Autodesk Inventor part; units mm, degrees
ref_plane "YZ Plane" through (0, 0, 0) normal (1, 0, 0) x (0, 1, 0)
ref_plane "XZ Plane" through (0, 0, 0) normal (0, 1, 0) x (-1, 0, 0)
ref_plane "XY Plane" through (0, 0, 0) normal (0, 0, 1) x (1, 0, 0)
sketch "スケッチ1" plane through (0, 0, 0) normal (0, 0, 1) x (1, 0, 0)
  line L0 (-20.6499, 10.2438) -> (19.8501, 10.2438)
  line L1 (19.8501, 10.2438) -> (19.8501, -10.7562)
  line L2 (19.8501, -10.7562) -> (-20.6499, -10.7562)
  line L3 (-20.6499, -10.7562) -> (-20.6499, 10.2438)
  dimension "d0" = 21
  dimension "d1" = 40.5
extrude "押し出し1" add sketch "スケッチ1" along normal blind 41.8
sketch "スケッチ2" plane through (0, 0, 41.8) normal (0, 0, 1) x (1, 0, 0)
  line L0 (-20.6499, 10.2438) -> (19.8501, 10.2438)
  line L1 (-20.6499, -10.7562) -> (-20.6499, 10.2438)
  line L2 (-13.3999, 16.2438) -> (12.6001, 16.2438)
  line L3 (12.6001, 16.2438) -> (12.6001, -16.7562)
  line L4 (12.6001, -16.7562) -> (-13.3999, -16.7562)
  line L5 (-13.3999, -16.7562) -> (-13.3999, 16.2438)
  line L6 (-13.3999, 12.7438) -> (12.6001, 12.7438)
  line L7 (12.6001, 12.7438) -> (12.6001, -13.2562)
  line L8 (12.6001, -13.2562) -> (-13.3999, -13.2562)
  line L9 (-13.3999, -13.2562) -> (-13.3999, 12.7438)
  circle A0 centre (-13.3999, 12.7438) radius 3.5
  circle A1 centre (-13.3999, -13.2562) radius 3.5
  circle A2 centre (12.6001, -13.2562) radius 3.5
  circle A3 centre (12.6001, 12.7438) radius 3.5
  line L10 (-16.8999, 12.7438) -> (-9.8999, 12.7438)
  line L11 (-9.8999, 12.7438) -> (-9.8999, -13.2562)
  line L12 (-9.8999, -13.2562) -> (-16.8999, -13.2562)
  line L13 (-16.8999, -13.2562) -> (-16.8999, 12.7438)
  line L14 (9.1001, 12.7438) -> (16.1001, 12.7438)
  line L15 (16.1001, 12.7438) -> (16.1001, -13.2562)
  line L16 (16.1001, -13.2562) -> (9.1001, -13.2562)
  line L17 (9.1001, -13.2562) -> (9.1001, 12.7438)
  dimension "d4" = 6
  dimension "d5" = 33
  dimension "d6" = 26
  dimension "d7" = 7.25
  dimension "d8" = 26
  dimension "d9" = 2.5
  dimension "d10" = 26
  dimension "d11" = 7
  dimension "d12" = 7
  dimension "d13" = 7
  dimension "d14" = 7
extrude "押し出し2" add sketch "スケッチ2" against normal blind 3.7 contours L13 A0 L0 | L0 A0 L5 A1 L13 | A0 L10 L5 L0 | L0 L5 A0 | L12 L5 A1 | A1 L5 L12 | A0 L5 L10 | L5 L6 A0 L0 | L0 A0 L5 | A0 L0 L11 A1 L5 | L5 L8 A1 | A1 L8 L5 | A0 L6 L5 | A0 L11 L0 | A2 L8 L3 | L3 L16 A2 | A3 L14 L3 | L3 L6 A3 | L8 A2 L3 | L3 A2 L16 | L17 L0 A3 L3 A2 | A2 L3 A3 L0 L15 | L14 A3 L0 L3 | L3 L0 A3 L6 | L15 L0 A3 | A3 L0 L17 | L3 A3 L0 | L0 A3 L3
sketch "スケッチ3" plane through (0, 0, 41.8) normal (0, 0, 1) x (1, 0, 0)
  line L0 (-20.6499, -10.7562) -> (-20.6499, 10.2438)
  line L1 (-9.8999, 10.2438) -> (9.1001, 10.2438)
  circle A0 centre (9.5501, -0.2562) radius 4
  dimension "d17" = 10.5
  dimension "d18" = 30.2
  dimension "d19" = 8
extrude "押し出し3" add sketch "スケッチ3" along normal blind 1.9
sketch "スケッチ4" plane through (9.5501, -0.2562, 43.7) normal (0, 0, 1) x (1, 0, 0)
  circle A0 centre (0, 0) radius 4
  circle A1 centre (0, 0) radius 10.5
  dimension "d22" = 21
extrude "押し出し4" add sketch "スケッチ4" along normal blind 1.9 contours A0 | A1
sketch "スケッチ5" plane through (9.5501, -0.2562, 45.6) normal (0, 0, 1) x (1, 0, 0)
  circle A0 centre (0, 0) radius 10.5
  circle A1 centre (0, 0) radius 4
  dimension "d25" = 8
extrude "押し出し5" add sketch "スケッチ5" along normal blind 1.2 contours A1
sketch "スケッチ6" plane through (9.5501, -0.2562, 46.8) normal (0, 0, 1) x (1, 0, 0)
  circle A0 centre (0, 0) radius 4
  circle A1 centre (0, 0) radius 2.75
  dimension "d28" = 5.5
extrude "押し出し6" add sketch "スケッチ6" along normal blind 3 contours A1
sketch "スケッチ7" plane through (0, 0, 0) normal (0, 0, -1) x (-1, 0, 0)
  line L0 (9.8999, -10.7562) -> (16.8999, -10.7562)
  line L1 (9.8999, -13.2562) -> (9.8999, -10.7562)
  arc A0 (9.8999, -13.2562) -> (16.8999, -13.2562) centre (13.3999, -13.2562) ccw
  line L2 (16.8999, -10.7562) -> (16.8999, -13.2562)
  line L3 (16.8999, 10.2438) -> (9.8999, 10.2438)
  line L4 (16.8999, 12.7438) -> (16.8999, 10.2438)
  arc A1 (16.8999, 12.7438) -> (9.8999, 12.7438) centre (13.3999, 12.7438) ccw
  line L5 (9.8999, 10.2438) -> (9.8999, 12.7438)
  line L6 (-9.1001, 10.2438) -> (-16.1001, 10.2438)
  line L7 (-9.1001, 12.7438) -> (-9.1001, 10.2438)
  arc A2 (-9.1001, 12.7438) -> (-16.1001, 12.7438) centre (-12.6001, 12.7438) ccw
  line L8 (-16.1001, 10.2438) -> (-16.1001, 12.7438)
  line L9 (-16.1001, -10.7562) -> (-9.1001, -10.7562)
  line L10 (-16.1001, -13.2562) -> (-16.1001, -10.7562)
  arc A3 (-16.1001, -13.2562) -> (-9.1001, -13.2562) centre (-12.6001, -13.2562) ccw
  line L11 (-9.1001, -10.7562) -> (-9.1001, -13.2562)
  line L12 (13.3999, -16.7562) -> (-12.6001, -16.7562)
  line L13 (-12.6001, -16.7562) -> (-12.6001, 16.2438)
  line L14 (-12.6001, 16.2438) -> (13.3999, 16.2438)
  line L15 (13.3999, 16.2438) -> (13.3999, -16.7562)
extrude "押し出し7" add sketch "スケッチ7" against normal blind 3.7
sketch "スケッチ8" plane through (0, 0, 0) normal (0, 0, -1) x (-1, 0, 0)
  line L0 (16.8999, -10.7562) -> (20.6499, -10.7562)
  line L1 (20.6499, -10.7562) -> (20.6499, 10.2438)
  line L2 (9.6499, -17.5562) -> (-8.8501, -17.5562)
  line L3 (-8.8501, -17.5562) -> (-8.8501, 17.0438)
  line L4 (-8.8501, 17.0438) -> (9.6499, 17.0438)
  line L5 (9.6499, 17.0438) -> (9.6499, -17.5562)
  dimension "d33" = 34.6
  dimension "d34" = 6.8
  dimension "d35" = 11
  dimension "d36" = 18.5
extrude "押し出し8" add sketch "スケッチ8" against normal blind 15
sketch "スケッチ9" plane through (19.8501, -10.7562, 0) normal (0, -1, 0) x (1, 0, 0)
  line L0 (-40.5, 0) -> (-40.5, 41.8)
  line L1 (-36.75, 0) -> (-40.5, 0)
  line L2 (-28.75, 31.6) -> (-11.75, 31.6)
  line L3 (-11.75, 31.6) -> (-11.75, 26.6)
  line L4 (-11.75, 26.6) -> (-28.75, 26.6)
  line L5 (-28.75, 26.6) -> (-28.75, 31.6)
  dimension "d39" = 26.6
  dimension "d40" = 5
  dimension "d41" = 11.75
  dimension "d42" = 17
extrude "押し出し9" add sketch "スケッチ9" along normal blind 6
sketch "スケッチ10" plane through (-20.6499, 10.2438, 41.8) normal (0, 1, 0) x (1, 0, 0)
  line L0 (28.75, 10.2) -> (28.75, 15.2)
  line L1 (11.75, 10.2) -> (28.75, 10.2)
  line L2 (11.75, 15.2) -> (11.75, 10.2)
  line L3 (28.75, 15.2) -> (11.75, 15.2)
extrude "押し出し10" add sketch "スケッチ10" along normal blind 6
fillet "フィレット1" radius 1 4 edges at (8.1001, -16.7562, 29.1) (-8.8999, -16.7562, 29.1) (8.1001, 16.2438, 29.1) (-8.8999, 16.2438, 29.1)
sketch "スケッチ11" plane through (-8.8999, -10.7562, 31.6) normal (0, 0, 1) x (1, 0, 0)
  line L0 (1, -6) -> (16, -6)
  line L1 (0, 0) -> (17, 0)
  line L2 (0, 0) -> (0, -5)
  line L3 (1, 0) -> (16, 0)
  line L4 (16, 0) -> (16, -4)
  line L5 (15, -5) -> (2, -5)
  line L6 (1, -4) -> (1, 0)
  line L7 (17, 0) -> (17, -5)
  arc A0 (1, -4) -> (2, -5) centre (2, -4) ccw
  arc A1 (15, -5) -> (16, -4) centre (15, -4) ccw
  arc A2 (17, 26) -> (16, 27) centre (16, 26) ccw
  line L8 (16, 27) -> (1, 27)
  arc A3 (1, 27) -> (0, 26) centre (1, 26) ccw
  line L9 (0, 21) -> (0, 26)
  line L10 (17, 21) -> (0, 21)
  line L11 (17, 21) -> (17, 26)
  line L12 (1, 21) -> (16, 21)
  line L13 (16, 21) -> (16, 25)
  line L14 (15, 26) -> (2, 26)
  line L15 (1, 25) -> (1, 21)
  arc A4 (2, 26) -> (1, 25) centre (2, 25) ccw
  arc A5 (16, 25) -> (15, 26) centre (15, 25) ccw
  dimension "d48" = 1
  dimension "d49" = 1
  dimension "d50" = 1
  dimension "d51" = 1
  dimension "d52" = 1
  dimension "d53" = 1
extrude "押し出し11" cut sketch "スケッチ11" against normal blind 6 contours L1 L4 A1 L5 A0 L6 | L10 L15 A4 L14 A5 L13
sketch "スケッチ12" plane through (0, 0, 41.8) normal (0, 0, 1) x (1, 0, 0)
  arc A0 (-16.8999, -13.2562) -> (-9.8999, -13.2562) centre (-13.3999, -13.2562) ccw
  arc A1 (9.1001, -13.2562) -> (16.1001, -13.2562) centre (12.6001, -13.2562) ccw
  arc A2 (16.1001, 12.7438) -> (9.1001, 12.7438) centre (12.6001, 12.7438) ccw
  arc A3 (-9.8999, 12.7438) -> (-16.8999, 12.7438) centre (-13.3999, 12.7438) ccw
hole "穴1" at (-13.3999, 12.7438, 41.8) at (12.6001, 12.7438, 41.8) at (12.6001, -13.2562, 41.8) at (-13.3999, -13.2562, 41.8) direction (0, 0, -1) diameter 2.2 depth 100 tip angle 118
chamfer "面取り1" distance 5 distance2 3 1 edges at (-20.6499, -0.2562, 41.8) measured on face at (-20.6499, -3.7562, 13.9333)
chamfer "面取り2" distance 5 distance2 3 1 edges at (19.8501, -0.2562, 41.8) measured on face at (19.8501, 3.2438, 13.9333)
sketch "スケッチ13" plane through (0, 0, 0) normal (0, 0, -1) x (-1, 0, 0)
  circle A0 centre (-9.5501, -0.2562) radius 4
hole "穴2" at (9.5501, -0.2562, 0) direction (0, 0, 1) diameter 2.459 depth 10 tip angle 118
sketch "スケッチ14" plane through (9.5501, -0.2562, 45.6) normal (0, 0, 1) x (1, 0, 0)
  circle A0 centre (0, 0) radius 4
  circle A1 centre (0, 0) radius 2.75
  circle A2 centre (0, 0) radius 7.5
  line L0 (0, 0) -> (7.5, 0)
  line L1 (0, 0) -> (6.9291, 2.8701)
  point P0 (2.8701, 6.9291)
  point P1 (-2.8701, 6.9291)
  point P2 (-6.9291, 2.8701)
  point P3 (-6.9291, -2.8701)
  point P4 (-2.8701, -6.9291)
  point P5 (2.8701, -6.9291)
  point P6 (6.9291, -2.8701)
  dimension "d76" = 15
  dimension "d77" = 22.5
  dimension "d80" = 360
hole "穴3" at (16.4792, 2.6139, 45.6) at (12.4202, 6.6729, 45.6) at (6.68, 6.6729, 45.6) at (2.621, 2.6139, 45.6) at (2.621, -3.1263, 45.6) at (6.68, -7.1853, 45.6) at (12.4202, -7.1853, 45.6) at (16.4792, -3.1263, 45.6) direction (0, 0, -1) diameter 1.567 depth 2 tip angle 118
properties part number "rs405"
Geometry: final body of the model. Coordinates: model frame, mm. A direction names the side the tool comes from. Give positions to 0.01 mm unless a question says otherwise; leave off trailing zeros. Write each loop counter-clockwise with the first axis right and the second up, starting at its lowest first coordinate (ties: lowest second). Pieces come first, ordered by that corner, then holes.
1. Draft query along Y for faces 1 (the flat face through (16.1, -12, 40)), 2 (the flat face through (0, -15.756, 29)), 3 (the flat face through (-1, -17.556, 7)). Return one class per face: released by +Y, released by -Y, zero draft, split by the parting line, or undercut.
2. Section query A-A, the plane y = 6.5. Return loops of the section in (x, z).
3. Section query D-D, the plane z = 21. Return loops of the section in (x, y), then the cut area to 4 significant figures.
4. Line query: probe 1 along X at (y, z) = (-11, 28); probe 2 along Z at (x, y) = (4, -8.5); probe 3 along X at (y, z) = (-5.5, 13). Output: solid intervals per line, ascending.
5. Reachability of faces 4 (the flat face through (18.329, -0.403, 39.335)), 5 (the cylindrical face through (-13.323, 16.243, 39.976)), 6 (the flat face through (8.1, -13, 29)) from +Z, -Z, +X, -X, +Y, -Y: full face, straight path, thin tool, end or side. Return the list, or none.
6. Pin query (flat end, axial travel): P1, Ø2.5, axis at x = 6.68, y = 6.67, coming from the +Z side; P2, Ø5, axis at x = 10.5, z = 36.5, coming from the -Y side; P3, Ø1.2, axis at y = 11, z = 2.5, coming from the -X side. Return the tip coordinate at first contact, or that it passes through.
7. Section query B-B, the plane x = 15. Return loops of the section in (y, z), then the cut area to 3 significant figures.
8. Section query C-C, the plane x = -15.5. Return loops of the section in (y, z).
Computed:
1. face 1: zero draft
1. face 2: undercut
1. face 3: released by -Y
2. outline: (-20.65, 0) - (19.85, 0) - (19.85, 36.8) - (16.85, 41.8) - (-17.65, 41.8) - (-20.65, 36.8) - close; (1.51, 43.7) - (5.92, 43.7) - (5.92, 45.6) - (1.51, 45.6) - close; (7.44, 43.7) - (11.66, 43.7) - (11.66, 45.6) - (7.44, 45.6) - close; (13.18, 43.7) - (17.59, 43.7) - (17.59, 45.6) - (13.18, 45.6) - close
3. outline: (-20.65, -10.76) - (19.85, -10.76) - (19.85, 10.24) - (-20.65, 10.24) - close
3. area: 850.5 mm2
4. probe 1: x = -8.9 to -7.9, 7.1 to 8.1
4. probe 2: z = 0 to 41.8, 43.7 to 45.6
4. probe 3: x = -20.65 to 19.85
5. face 4: +X, +Y, -Y
5. face 5: +Z, +Y
5. face 6: +Z, +X, -Y
6. P1: stops at z = 45.6
6. P2: stops at y = -16.75
6. P3: stops at x = -16.9
7. outline: (-15.8, 0) - (15.29, 0) - (15.29, 3.7) - (10.24, 3.7) - (10.24, 38.1) - (15.29, 38.1) - (15.29, 41.8) - (-15.8, 41.8) - (-15.8, 38.1) - (-10.76, 38.1) - (-10.76, 3.7) - (-15.8, 3.7) - close; (-9.23, 43.7) - (8.72, 43.7) - (8.72, 45.6) - (-9.23, 45.6) - close
7. area: 987 mm2
8. outline: (-16.06, 0) - (15.54, 0) - (15.54, 3.7) - (10.24, 3.7) - (10.24, 38.1) - (15.54, 38.1) - (15.54, 41.8) - (-16.06, 41.8) - (-16.06, 38.1) - (-10.76, 38.1) - (-10.76, 3.7) - (-16.06, 3.7) - close
